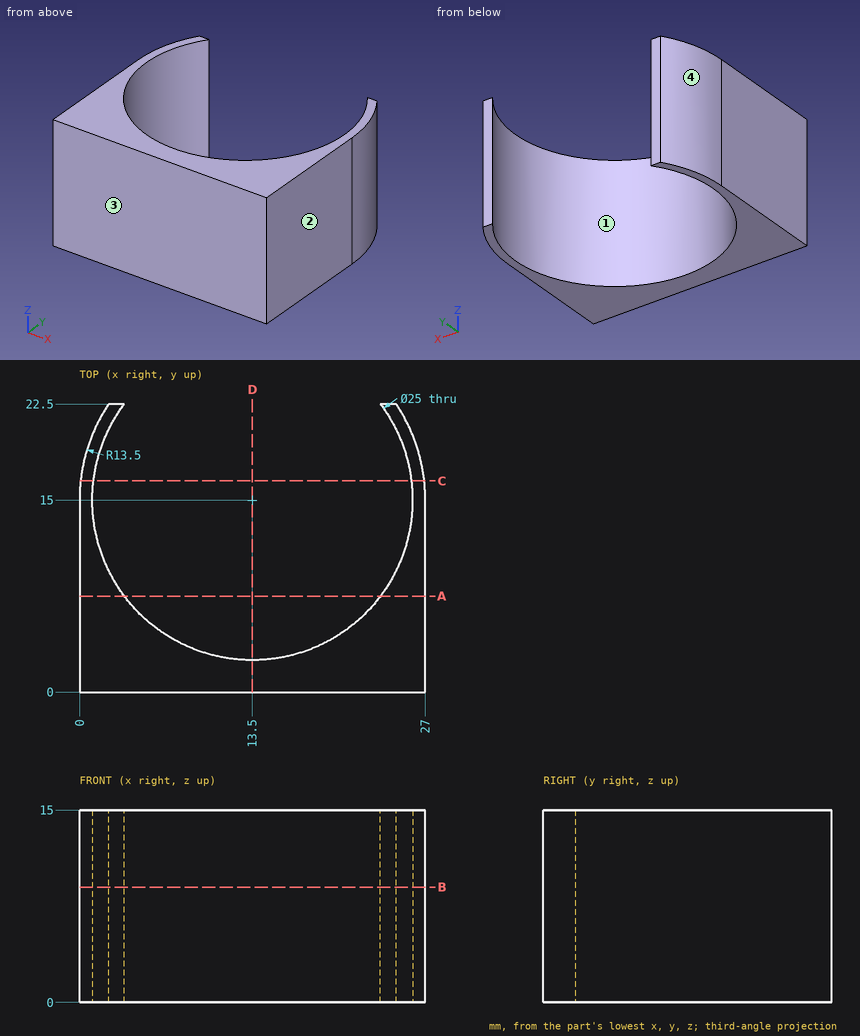
Part print with two shaded views. Sizes in mm from the minimum x, y, z corner. Give positions to 0.01 mm unless a question says otherwise; leave off trailing zeros. Order: outer loops, then holes, each group sorted by start corner. A loop starts at its lowest first (then second) coordinate and runs counter-clockwise, first axis right, second up. Notation, with made-up numbers: M 47,86 L 54,86 A7 ccw 54,97 Z; hole C 60.5,-10 d11. An arc over 180 degrees is marked long. Put each result on its own line as item: value.
Item 1: Cut at B-B on z = 9. Write the cut outline in (x, y), then the cut area to 3 significant figures.
Results are:
outline: M 0,0 L 27,0 L 27,15 A13.5 ccw 24.72,22.5 L 23.5,22.5 A12.5 cw long 3.5,22.5 L 2.28,22.5 A13.5 ccw 0,15 Z
area: 176 mm2
Item 2: Cut at D-D on x = 13.5. Write the cut outline in (y, z), then the cut area to 3 significant figures.
Results are:
outline: M 0,0 L 2.5,0 L 2.5,15 L 0,15 Z
area: 37.5 mm2
Item 3: Pull direction Y, two halves, no side cores. Call the marked faces 1, 2, 3 and 4: +Y half, -Y half, draft (parallel to the pull), parting line (faces both ways), or undercut.
Results are:
face 1: undercut
face 2: draft
face 3: -Y half
face 4: +Y half
Item 4: Cut at A-A on y = 7.5. Write the cut outline in (x, z), then the cut area to 3 significant figures.
Results are:
outline: M 0,0 L 3.5,0 L 3.5,15 L 0,15 Z; M 23.5,0 L 27,0 L 27,15 L 23.5,15 Z
area: 105 mm2
Item 5: Wall check: probe 1 along X at (y, z) = (15, 3.5); probe 2 along X at (y, z) = (11.5, 1.25); probe 3 along Y at (x, z) = (10.5, 10.25). Give the ranges that are in metal, low to high.
Results are:
probe 1: 0 to 1, 26 to 27
probe 2: 0 to 1.5, 25.5 to 27
probe 3: 0 to 2.87
Item 6: Cut at C-C on y = 16.5. Write the cut outline in (x, z).
Results are:
outline: M 0.08,0 L 1.09,0 L 1.09,15 L 0.08,15 Z; M 25.91,0 L 26.92,0 L 26.92,15 L 25.91,15 Z
